from build123d import *

# Parameters (mm, degrees)
SKETCH_1_R      = 16
EXTRUDE_1_DEPTH = 15
SKETCH_2_R      = 45
SKETCH_2_R_2    = 12
EXTRUDE_3_DEPTH = 3
SKETCH_3_R      = 55
SKETCH_3_R_2    = 45
EXTRUDE_4_DEPTH = 11


with BuildPart() as part:
    # 草图1 → 凸台-拉伸1 (new, symmetric)
    with BuildSketch(Plane(origin=(0, 0, 0), x_dir=(1, 0, 0), z_dir=(0, 1, 0))):
        with Locations(Location((0, 0, 0), (0, 0, 270))):
            Circle(SKETCH_1_R)
        with BuildLine():
            ThreePointArc((2, 7.228416147), (0, -7.5), (-2, 7.228416147))
            Line((-2, 7.228416147), (-2, 9.6))
            Line((-2, 9.6), (2, 9.6))
            Line((2, 9.6), (2, 7.228416147))
        make_face(mode=Mode.SUBTRACT)
    extrude(amount=EXTRUDE_1_DEPTH, both=True)

    # 草图2 → 凸台-拉伸3 (add, symmetric)
    with BuildSketch(Plane(origin=(0, 0, 0), x_dir=(1, 0, 0), z_dir=(0, 1, 0))):
        with Locations(Location((0, 0, 0), (0, 0, 270))):
            Circle(SKETCH_2_R)
        with Locations(Location((-30, 0, 0), (0, 0, 270))):
            Circle(SKETCH_2_R_2, mode=Mode.SUBTRACT)
        with Locations(Location((-15, 25.980762114, 0), (0, 0, 270))):
            Circle(SKETCH_2_R_2, mode=Mode.SUBTRACT)
        with Locations(Location((15, 25.980762114, 0), (0, 0, 270))):
            Circle(SKETCH_2_R_2, mode=Mode.SUBTRACT)
        with Locations(Location((30, 0, 0), (0, 0, 270))):
            Circle(SKETCH_2_R_2, mode=Mode.SUBTRACT)
        with Locations(Location((15, -25.980762114, 0), (0, 0, 270))):
            Circle(SKETCH_2_R_2, mode=Mode.SUBTRACT)
        with Locations(Location((-15, -25.980762114, 0), (0, 0, 270))):
            Circle(SKETCH_2_R_2, mode=Mode.SUBTRACT)
    extrude(amount=EXTRUDE_3_DEPTH, both=True)

    # 草图3 → 凸台-拉伸4 (add, symmetric)
    with BuildSketch(Plane(origin=(0, 0, 0), x_dir=(1, 0, 0), z_dir=(0, 1, 0))):
        with Locations(Location((0, 0, 0), (0, 0, 270))):
            Circle(SKETCH_3_R)
        with Locations(Location((0, 0, 0), (0, 0, 270))):
            Circle(SKETCH_3_R_2, mode=Mode.SUBTRACT)
    extrude(amount=EXTRUDE_4_DEPTH, both=True)

    # 草图4 → 切除-旋转1 (revolve, cut)
    with BuildSketch(Plane.XY, mode=Mode.PRIVATE) as cut_revolve_1_sk:
        Polygon((-55, 1.5), (-50, 3.221638066), (-50, 5.263530397), (-55, 6.985168464), align=None)
        Polygon((-55, -1.5), (-50, -3.221638066), (-50, -5.263530397), (-55, -6.985168464), align=None)
    revolve(cut_revolve_1_sk.sketch.rotate(Axis((0, -16.5, 0), (0, 1, 0)), 270), axis=Axis((0, -16.5, 0), (0, 1, 0)), mode=Mode.SUBTRACT)


solid = part.part
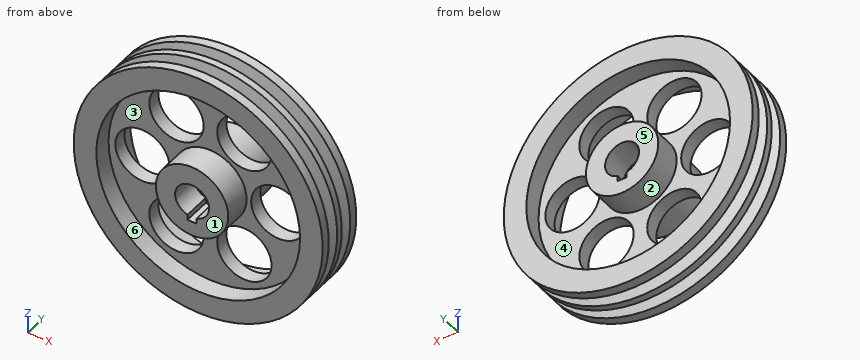
CAD build for the part. Positions are in the model's coordinates, mm. Face numbers are marked on the shaded views. A direction names the side the tool comes from. Round coordinates to 2 decimals unless told otherwise and drop trailing zeros. Write each loop counter-clockwise with the first axis right and the second up, starting at its lowest first coordinate (ties: lowest second). Pieces come first, ordered by that corner, then holes. Notation, with made-up numbers: (70.5, 72) -> (118.5, 72) arc R6 ccw to (118.5, 80) -> close; hole circle Ø8 at (-37, 53.25). An arc over 180 degrees is marked (long way). Answer as a JSON object with one key per item and string values.
(1) Probe probe 1 along X at (y, z) = (-0.3, 0); probe 2 along X at (y, z) = (0, -28); probe 3 along X at (y, z) = (8.25, 0). List the from-to ranges inside material, lowest first. Write a range as [from, to].
Reported:
{"probe 1": "x = [-55, -42], [-18, 18], [42, 55]", "probe 2": "x = [-47.34, -26.83], [-3.17, 3.17], [26.83, 47.34]", "probe 3": "x = [-55, -45], [-16, -7.5], [7.5, 16], [45, 55]"}
(2) Band-saw the part on B-B, the plane z = 0. Count the separate pieces of the cut face and the enclosed holes in it, then the cut area to 3 significant figures.
Reported:
{"separate pieces": "3", "enclosed holes": "0", "area": "1,020 mm^2"}
(3) Which spindle directions (+Z, -Z, +X, -X, +Y, -Y) get a long thin tool onto all of the face, cutting with end or side? Do the marked faces 1, 2 and 3. Say none if no direction does.
Reported:
{"face 1": "+Z, -Z, +X, -X, -Y", "face 2": "+Y", "face 3": "-Y"}
(4) Two-plate mould, pull along Z, no slides. Class the marked faces 4, 5 and 6: +Z half, -Z half, draft (parallel to the pull), parting line (faces both ways), or undercut.
Reported:
{"face 4": "undercut", "face 5": "draft", "face 6": "undercut"}
(5) Pin check, flat tips, straight feed: P1, Ø8, axis at y = -9, z = -36.5, coming from the -X side; P2, Ø5, axis at x = -2, z = 41, coming from the -Y side; P3, Ø19, axis at x = 15, z = 25.98, coming from the -Y side; P4, Ø5, axis at y = -5.5, z = -31.5, coming from the -X side. Stop position of each tip, or through.
Reported:
{"P1": "stops at x = -44.37", "P2": "stops at y = -3", "P3": "passes through", "P4": "stops at x = -46.43"}
(6) Band-saw the part on A-A, the plane y = 8.75. List the corners of the cut face in (x, z).
Reported:
{"outline": "circle Ø110 at (0, 0); circle Ø32 at (0, 0); hole circle Ø90 at (0, 0); hole (-2, -9.6) -> (2, -9.6) -> (2, -7.23) arc R7.5 ccw (long way) to (-2, -7.23) -> close"}
